```python
from build123d import *

# Parameters (mm, degrees)
SKETCH1_W           = 55.99
SKETCH1_H           = 87.9
SKETCH1_R           = 3.5
BOSS_EXTRUDE1_DEPTH = 10
FILLET1_R           = 8
FILLET2_R           = 1
CHAMFER1_SIZE       = 0.5


# Read off the part's stored shape, not the designer's step: Split1
with BuildPart() as part:
    # Sketch1 → Boss-Extrude1 (new body)
    with BuildSketch(Plane.XY):
        with Locations((-17.995, 31.45)):
            Rectangle(SKETCH1_W, SKETCH1_H)
        Circle(SKETCH1_R, mode=Mode.SUBTRACT)
        with Locations((-6.59, 32)):
            Circle(SKETCH1_R, mode=Mode.SUBTRACT)
        with Locations((-20.59, 32)):
            Circle(SKETCH1_R, mode=Mode.SUBTRACT)
        with Locations((-14, 0)):
            Circle(SKETCH1_R, mode=Mode.SUBTRACT)
        with Locations((-20.59, 50)):
            Circle(SKETCH1_R, mode=Mode.SUBTRACT)
        with Locations((-20.59, 68)):
            Circle(SKETCH1_R, mode=Mode.SUBTRACT)
        with Locations((-38.59, 68)):
            Circle(SKETCH1_R, mode=Mode.SUBTRACT)
        with Locations((-38.59, 50)):
            Circle(SKETCH1_R, mode=Mode.SUBTRACT)
    extrude(amount=BOSS_EXTRUDE1_DEPTH)

    # Fillet1
    fillet1_edges = [part.edges().sort_by_distance(p)[0] for p in [
        (-45.99, -12.5, 5),
        (-45.99, 75.4, 5),
        (10, 75.4, 5),
        (10, -12.5, 5),
    ]]
    fillet(fillet1_edges, radius=FILLET1_R)


with BuildPart() as body_2:
    # Split1: the piece on the far side of the plane
    add(part.part)
    split(bisect_by=Plane(origin=(0, 41, 0), x_dir=(1, 0, 0), z_dir=(0, 1, 0)), keep=Keep.BOTTOM)


with BuildPart() as part_1:
    add(part.part)

    # Split1
    split(bisect_by=Plane(origin=(0, 41, 0), x_dir=(1, 0, 0), z_dir=(0, 1, 0)), keep=Keep.TOP)

    # Fillet2
    fillet2_edges = [part_1.edges().sort_by_distance(p)[0] for p in [
        (-17.995, 41, 0),
        (-45.99, 54.2, 0),
        (-17.995, 75.4, 0),
        (7.656854249, 73.056854249, 0),
        (-43.646854249, 73.056854249, 0),
        (-17.995, 75.4, 10),
        (-45.99, 54.2, 10),
        (7.656854249, 73.056854249, 10),
        (-43.646854249, 73.056854249, 10),
        (-45.99, 41, 5),
        (10, 54.2, 10),
        (10, 54.2, 0),
        (10, 41, 5),
        (-17.995, 41, 10),
    ]]
    fillet(fillet2_edges, radius=FILLET2_R)

    # Chamfer1
    chamfer1_edges = [part_1.edges().sort_by_distance(p)[0] for p in [
        (-24.09, 50, 0),
        (-24.09, 50, 10),
        (-24.09, 68, 0),
        (-24.09, 68, 10),
        (-42.09, 68, 0),
        (-42.09, 68, 10),
        (-42.09, 50, 0),
        (-42.09, 50, 10),
    ]]
    chamfer(chamfer1_edges, length=CHAMFER1_SIZE)


solid = part_1.part
```
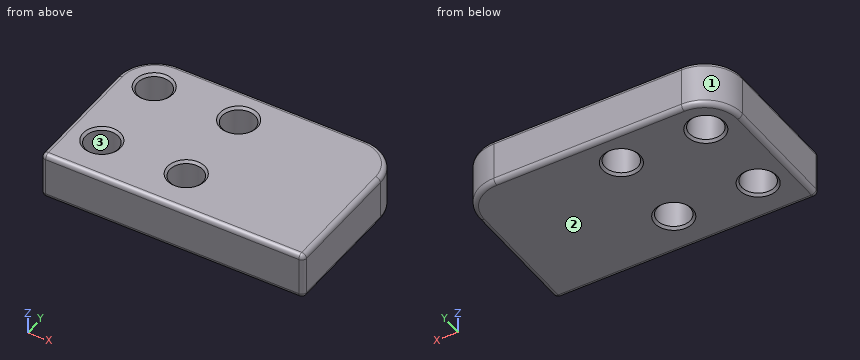
Build history of the part. All positions in model axes, mm. Face numbers are marked on the shaded views. Coordinates: 2 decimals unless noted, no trailing zeros. Order: outer loops, then holes, each group sorted by start corner. A loop starts at its lowest first (then second) coordinate and runs counter-clockwise, first axis right, second up.
Item 1: Saw through at B-B on z = 5. List the corners of the cut face in (x, y).
Filled in:
outline: (-45.99, 42) arc R1 ccw to (-44.99, 41) - (9, 41) arc R1 ccw to (10, 42) - (10, 67.4) arc R8 ccw to (2, 75.4) - (-37.99, 75.4) arc R8 ccw to (-45.99, 67.4) - close; hole circle Ø7 at (-38.59, 50); hole circle Ø7 at (-38.59, 68); hole circle Ø7 at (-20.59, 50); hole circle Ø7 at (-20.59, 68)
Item 2: Saw through at C-C on x = -39. State how many separate pieces and enclosed holes the cut face has, then the cut area to 3 significant figures.
Filled in:
separate pieces: 3
enclosed holes: 0
area: 202 mm2
Item 3: Drill centre lines: L1, parallel to Y at x = -20.59, z = 6.5; L2, parallel to X at y = 68.5, z = 6; L3, parallel to X at y = 49, z = 2. Where is each one in solid material? Low to high.
Filled in:
L1: y = 41 to 46.5, 53.5 to 64.5, 71.5 to 75.4
L2: x = -45.91 to -42.05, -35.13 to -24.05, -17.13 to 9.92
L3: x = -45.99 to -41.94, -35.24 to -23.94, -17.24 to 10
Item 4: Saw through at A-A on y = 50. List the corners of the cut face in (x, z), then the cut area to 3 significant figures.
Filled in:
outline: (-45.99, 1) arc R1 ccw to (-44.99, 0) - (-42.59, 0) - (-42.09, 0.5) - (-42.09, 9.5) - (-42.59, 10) - (-44.99, 10) arc R1 ccw to (-45.99, 9) - close; (-35.09, 0.5) - (-34.59, 0) - (-24.59, 0) - (-24.09, 0.5) - (-24.09, 9.5) - (-24.59, 10) - (-34.59, 10) - (-35.09, 9.5) - close; (-17.09, 0.5) - (-16.59, 0) - (9, 0) arc R1 ccw to (10, 1) - (10, 9) arc R1 ccw to (9, 10) - (-16.59, 10) - (-17.09, 9.5) - close
area: 418 mm2
Item 5: Mould opens along X. For the marked faces 1, 2 and 3 say: released by +X, released by -X, zero draft, split by the parting line, or undercut.
Filled in:
face 1: released by -X
face 2: zero draft
face 3: undercut
Item 6: Drop a flat-ended pin along its axis: pin 1 Ø6 at (y, z) = (71.5, 6) entering from -X. Give the stop position or say it passes through.
Filled in:
pin 1: stops at x = -45.91
